Autodesk Inventor part; units mm, degrees
ref_plane "YZ Plane" through (0, 0, 0) normal (1, 0, 0) x (0, 1, 0)
ref_plane "XZ Plane" through (0, 0, 0) normal (0, 1, 0) x (-1, 0, 0)
ref_plane "XY Plane" through (0, 0, 0) normal (0, 0, 1) x (1, 0, 0)
sketch "Boceto1" plane through (0, 0, 0) normal (0, 1, 0) x (-1, 0, 0)
  line L0 (10.3005, 0.2018) -> (-1.6995, 0.2018)
  line L1 (-1.6995, 0.2018) -> (-1.6995, 18.2018)
  line L2 (-1.6995, 18.2018) -> (10.3005, 18.2018)
  line L3 (12.3005, 20.2018) -> (-3.6995, 20.2018)
  line L4 (-3.6995, 20.2018) -> (-3.6995, -1.7982)
  line L5 (-3.6995, -1.7982) -> (12.3005, -1.7982)
  line L6 (10.3005, 18.2018) -> (12.3005, 18.2018)
  line L7 (10.3005, 0.2018) -> (12.3005, 0.2018)
  line L8 (12.3005, -1.7982) -> (12.3005, 0.2018)
  line L9 (12.3005, 18.2018) -> (12.3005, 20.2018)
  point P0 (0, 0)
  point P1 (0, 0)
  dimension "d0" = 18
  dimension "d1" = 12
extrude "Extrusión1" add sketch "Boceto1" along normal blind 28
sketch "Boceto2" plane through (-12.3005, 0, 20.2018) normal (0, 0, 1) x (1, 0, 0)
  line L0 (0, 0) -> (0, 1.5)
  line L1 (0, 0) -> (0, 28)
  line L2 (0, 0) -> (14, 0)
  line L3 (16, 0) -> (16, 28)
  line L4 (0, 0) -> (16, 0)
  line L5 (16, 0) -> (16, 1.5)
  arc A0 (16, 1.5) -> (0, 1.5) centre (8, 1.5) ccw
  circle A1 centre (8, 5) radius 1.75
  point P0 (12.3005, 0)
  dimension "d4" = 1.5
  dimension "d5" = 3.5
  dimension "d6" = 5
extrude "Extrusión2" cut sketch "Boceto2" against normal blind 1
sketch "Boceto3" plane through (3.6995, 0, -1.7982) normal (0, 0, -1) x (-1, 0, 0)
  line L0 (0, 0) -> (0, 1.5)
  line L1 (0, 0) -> (0, 25)
  line L2 (0, 0) -> (14, 0)
  line L3 (16, 0) -> (16, 25)
  line L4 (0, 0) -> (16, 0)
  line L5 (16, 0) -> (16, 1.5)
  arc A0 (16, 1.5) -> (0, 1.5) centre (8, 1.5) ccw
  circle A1 centre (8, 5) radius 1.75
  point P0 (3.6995, 0)
  point P1 (12.3005, 0)
  dimension "d9" = 1.5
  dimension "d10" = 3.5
  dimension "d11" = 5
extrude "Extrusión3" cut sketch "Boceto3" against normal blind 1
sketch "Boceto4" plane through (1.6995, 0, 0.2018) normal (-1, 0, 0) x (0, 0, 1)
  line L0 (18, 0) -> (18, 28)
  line L1 (18, 28) -> (18, 12)
  line L2 (18, 12) -> (0, 12)
  line L3 (0, 0) -> (0, 28)
  line L4 (18, 28) -> (0, 28)
  line L5 (0, 28) -> (0, 12)
  line L6 (20, 28) -> (-2, 28)
  line L7 (9, 28) -> (9, 12)
  circle A0 centre (9, 24) radius 1.75
  circle A1 centre (9, 16) radius 1.75
  line L8 (18, 12) -> (18, 0)
  line L9 (0, 0) -> (18, 0)
  line L10 (0, 0) -> (0, 12)
  line L11 (18, 0) -> (0, 0)
  point P0 (-0.2018, 0)
  dimension "d14" = 16
  dimension "d15" = 3.5
  dimension "d16" = 3.5
  dimension "d17" = 4
  dimension "d18" = 4
extrude "Extrusión4" cut sketch "Boceto4" against normal blind 2 contours L9 L3 L2 L0 | A1 L7 | L7 A1 | A0 L7 | L7 A0
sketch "Boceto5" plane through (3.6995, 28, -1.7982) normal (0, 0, -1) x (-1, 0, 0)
  line L0 (0, -26.5) -> (0, 0)
  line L1 (0, 0) -> (4, 0)
  line L2 (16, 0) -> (0, 0)
  line L3 (0, 0) -> (0, -16)
  line L4 (0, -16) -> (16, -16)
  line L5 (16, -26.5) -> (16, 0)
  line L6 (4, 0) -> (16, -16)
  line L7 (4, 0) -> (4, -16)
  point P0 (3.6995, -28)
  dimension "d21" = 4
  dimension "d22" = 16
extrude "Extrusión5" cut sketch "Boceto5" against normal blind 30 contours L2 L5 L6
properties part number "Kit de Sujeción 1"
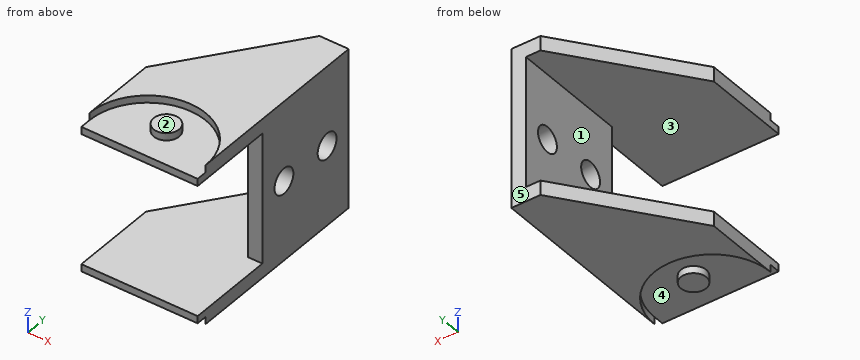
The listing builds one solid part. Answer for the finished solid, in the listing's coordinates (mm). Face numbers are marked on the shaded views. A direction names the side the tool comes from. Coordinates: 2 decimals unless noted, no trailing zeros. Loops run counter-clockwise (first coordinate to the right, second up) from the corner with the lowest first, then second, coordinate; pieces in that order, holes last. Notation, with made-up numbers: (-30.75, -34) -> (23.25, -34) arc R6 ccw to (23.25, -24) -> close; hole circle Ø8 at (73.5, 36.25). An arc over 180 degrees is marked (long way). Answer in a Markdown table with one row per item. Add a question column.
1. For the marked faces 1 and 2, determine the directions among +Z, -Z, +X, -X, +Y, -Y from which every point of the face is accessible in a straight line to the end or side of a thin tool.
2. Flat-ended cylindrical pins translate along their axes: P1, Ø1, axis at x = 3, z = 10.5, coming from the -Y side; P2, Ø1.5, axis at y = 8.5, z = 17.5, coming from the -X side; P3, Ø4.5, axis at y = 16, z = 9.2, coming from the -X side. Find the tip coordinate at first contact, or state that the pin passes through.
3. The part is cut by section A-A, the plane y = 11.5. Write down the section's boundary in (x, z), then the cut area to 3 significant figures.
4. The part is cut by section C-C, the plane z = 8. Write down the section's boundary in (x, y).
5. The part is cut by section D-D, the plane y = 8.5. Write down the section's boundary in (x, z).
6. The part is cut by section B-B, the plane x = -3.75. Write down the section's boundary in (y, z).
7. Determine the mould class of the marked faces 3, 4 and 5 for opening direction Z: +Z half, -Z half, draft (parallel to the pull), parting line (faces both ways), or undercut.
8. Consider line 1 (Z direction, x = 2.6, y = 16); line 2 (Z direction, x = -5.75, y = 18.25); line 3 (X direction, y = 25.75, z = 2). Determine where each line is inside the solid, lowest interval first. Write a range as [from, to].
Answer below:
| question | item | result |
|---|---|---|
| 1 | face 1 | -X, +Y, -Y |
| 1 | face 2 | +Z, +X, -X, +Y, -Y |
| 2 | P1 | y = 12 |
| 2 | P2 | x = -12.3 |
| 2 | P3 | x = 1.7 |
| 3 | outline | (-12.3, -1.8) -> (3.7, -1.8) -> (3.7, 0.2) -> (-12.3, 0.2) -> close; (-12.3, 18.2) -> (3.7, 18.2) -> (3.7, 20.2) -> (-12.3, 20.2) -> close |
| 3 | area | 64.0 mm2 |
| 4 | outline | (1.7, 12) -> (3.7, 12) -> (3.7, 14.73) -> (1.7, 14.73) -> close; (1.7, 17.27) -> (3.7, 17.27) -> (3.7, 22.73) -> (1.7, 22.73) -> close; (1.7, 25.27) -> (3.7, 25.27) -> (3.7, 28) -> (1.7, 28) -> close |
| 5 | outline | (-12.3, -1.8) -> (-8.17, -1.8) -> (-8.17, -0.8) -> (-0.43, -0.8) -> (-0.43, -1.8) -> (3.7, -1.8) -> (3.7, 0.2) -> (-12.3, 0.2) -> close; (-12.3, 18.2) -> (3.7, 18.2) -> (3.7, 20.2) -> (-0.43, 20.2) -> (-0.43, 19.2) -> (-8.17, 19.2) -> (-8.17, 20.2) -> (-12.3, 20.2) -> close |
| 6 | outline | (0, -0.8) -> (3.34, -0.8) -> (3.34, -1.8) -> (6.66, -1.8) -> (6.66, -0.8) -> (9.48, -0.8) -> (9.48, -1.8) -> (23.4, -1.8) -> (23.4, 0.2) -> (0, 0.2) -> close; (0, 18.2) -> (23.4, 18.2) -> (23.4, 20.2) -> (9.48, 20.2) -> (9.48, 19.2) -> (6.66, 19.2) -> (6.66, 20.2) -> (3.34, 20.2) -> (3.34, 19.2) -> (0, 19.2) -> close |
| 7 | face 3 | undercut |
| 7 | face 4 | -Z half |
| 7 | face 5 | draft |
| 8 | line 1 | [-1.8, 7.45], [10.95, 20.2] |
| 8 | line 2 | [-1.8, 0.2], [18.2, 20.2] |
| 8 | line 3 | [1.7, 3.7] |
